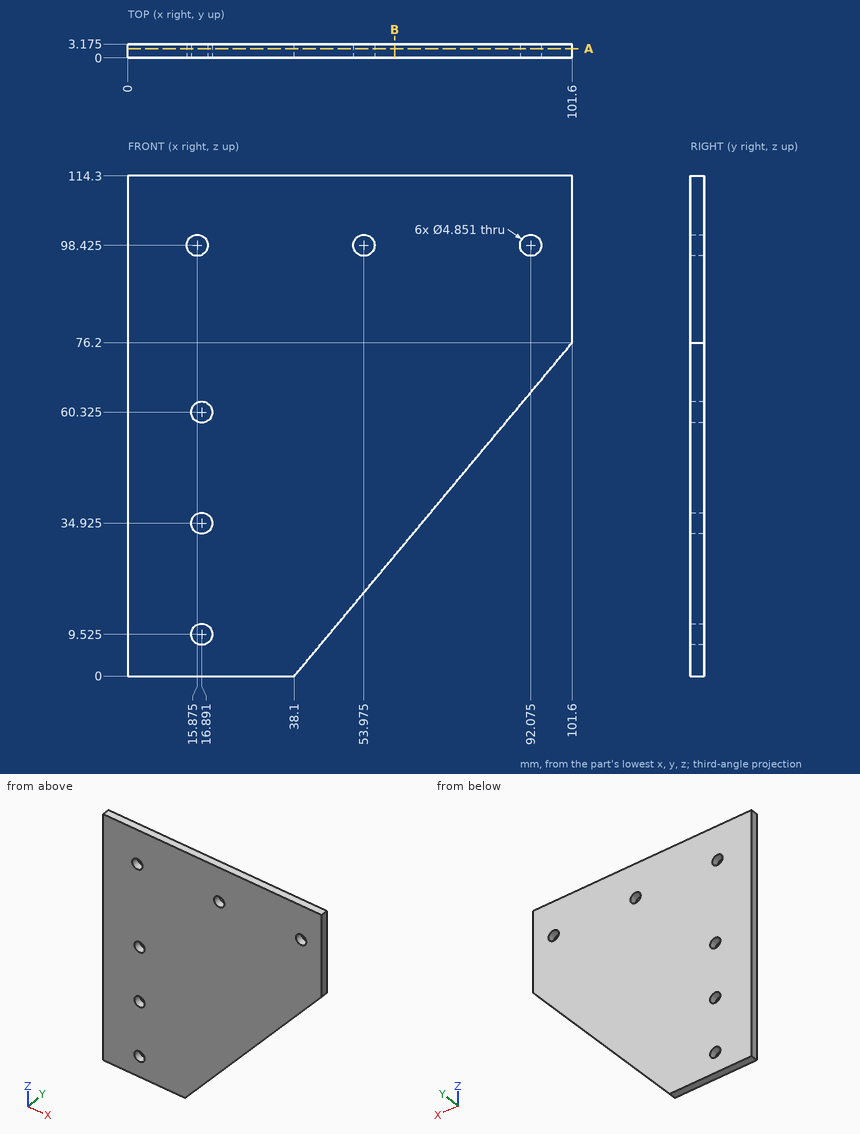
Answer from the drawing. Dimensions are ordinates in mm from the lowest x, y and z of the part. Give positions to 0.01 mm unless a question says otherwise; leave off trailing zeros. Write each loop counter-clockwise with the first axis right and the second up, starting at its lowest first coordinate (ties: lowest second). Pieces come first, ordered by that corner, then holes. Notation, with made-up numbers: (-21.5, 35.25) - (-7.5, 35.25) arc R24 ccw to (-7.5, 54.25) - close; hole circle Ø2 at (54, -19.75). An arc over 180 degrees is marked (long way). Answer in a Markdown table with one row per item. Add a question column.
Item 1: Flat-ended cylindrical pins translate along their axes: P1, Ø4.5, axis at x = 15.875, z = 98.425, coming from the -Y side; P2, Ø6.5, axis at x = 16.891, z = 34.925, coming from the -Y side; P3, Ø1, axis at y = 1.5, z = 30, coming from the +X side; P4, Ø1, axis at x = 50, y = 1, coming from the -Z side. Find the tip coordinate at first contact, or state that the pin passes through.
Item 2: Find the intervals of material crossed by L1, parallel to X at y = 2.65, z = 100; L2, parallel to X at y = 0.85, z = 33 (1 decimal); L3, parallel to X at y = 0.8, z = 46.5, in increasing order.
Item 3: Section A-A, the plane y = 2.1 is taken. Count the separate pieces of the cut face and the enclosed holes in it, and give its area (3 significant figures).
Item 4: Section B-B, the plane x = 61 is taken. Write down the section's boundary in (y, z) (1 decimal), and give its area (3 significant figures).
Recorded:
| question | item | result |
|---|---|---|
| 1 | P1 | passes through |
| 1 | P2 | stops at y = 0 |
| 1 | P3 | stops at x = 63.52 |
| 1 | P4 | stops at z = 13.68 |
| 2 | L1 | x = 0 to 14.03, 17.72 to 52.13, 55.82 to 90.23, 93.92 to 101.6 |
| 2 | L2 | x = 0 to 15.4, 18.4 to 65.6 |
| 2 | L3 | x = 0 to 76.85 |
| 3 | separate pieces | 1 |
| 3 | enclosed holes | 6 |
| 3 | area | 9,080 mm2 |
| 4 | outline | (0, 27.5) - (3.2, 27.5) - (3.2, 114.3) - (0, 114.3) - close |
| 4 | area | 276 mm2 |
